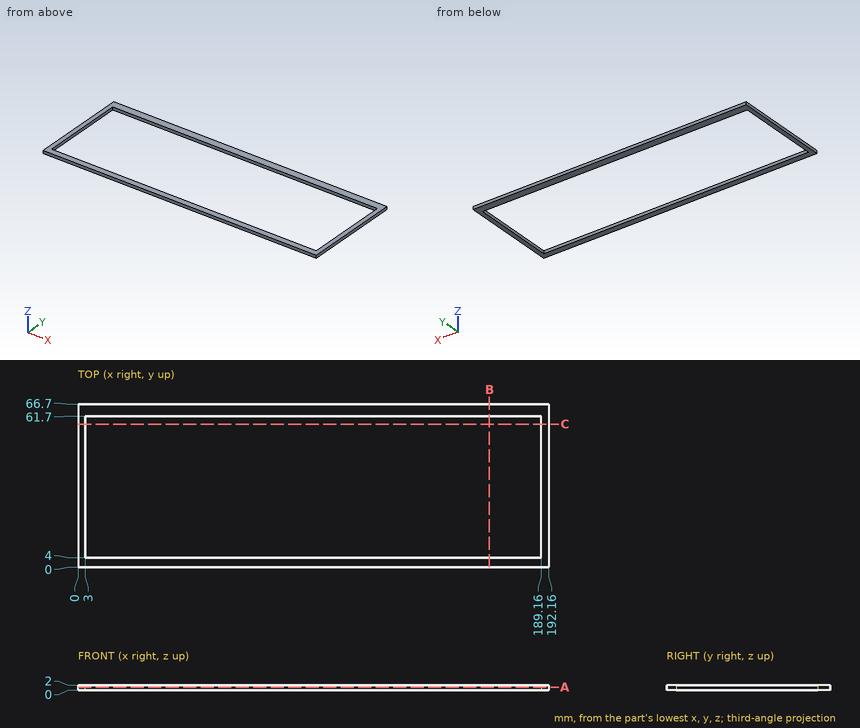
For this review, use the dimensioned drawing (mm, ordinates from the lowest corner) and the shaded views. Coordinates: 2 decimals unless noted, no trailing zeros. Order: outer loops, then holes, each group sorted by start corner. A loop starts at its lowest first (then second) coordinate and runs counter-clockwise, first axis right, second up. Notation, with made-up numbers: (77, -31.75) -> (82, -31.75) arc R19 ccw to (82, -17.75) -> close; hole circle Ø1 at (34, 32.25). An arc over 180 degrees is marked (long way). One line per item, written item: value. Start each with the question number.
Q1. Take a section at B-B, the plane x = 168. State the section outline as (y, z) points.
Q2. Take a section at C-C, the plane y = 58.5. State the section outline as (x, z) points, then the cut area to 3 significant figures.
Q3. Take a section at A-A, the plane z = 1.3. State the section outline as (x, y) points, then the cut area to 3 significant figures.
Q4. For probe 1 along Y at (x, z) = (171, 1.6); probe 2 along X at (y, z) = (10, 1.9), list the stretches that pass through material, from the lowest coordinate up.
Values follow:
1. outline: (0, 0) -> (4, 0) -> (4, 2) -> (0, 2) -> close; (61.7, 0) -> (66.7, 0) -> (66.7, 2) -> (61.7, 2) -> close
2. outline: (0, 0) -> (3, 0) -> (3, 2) -> (0, 2) -> close; (189.16, 0) -> (192.16, 0) -> (192.16, 2) -> (189.16, 2) -> close
2. area: 12.0 mm2
3. outline: (0, 0) -> (192.16, 0) -> (192.16, 66.7) -> (0, 66.7) -> close; hole (3, 4) -> (189.16, 4) -> (189.16, 61.7) -> (3, 61.7) -> close
3. area: 2,080 mm2
4. probe 1: y = 0 to 4, 61.7 to 66.7
4. probe 2: x = 0 to 3, 189.16 to 192.16
